Work out the finished part from the listing and answer in its coordinate system (mm). A direction names the side the tool comes from. Round coordinates to 2 decimals unless told otherwise and drop trailing zeros. Order: outer loops, then holes, each group sorted by start corner. A loop starts at its lowest first (then second) coordinate and runs counter-clockwise, first axis right, second up. Notation, with made-up numbers: (8.25, 79.5) - (46.25, 79.5) arc R26 cw to (46.25, 93.5) - close; hole circle Ø2 at (-9, -38.75). An arc over 180 degrees is marked (long way). Use CSV: the item, a comma, the result in double quotes.
from build123d import *

# Parameters (mm, degrees)
BOSS_EXTRUDE1_START = 1
SKETCH1_R           = 20
BOSS_EXTRUDE1_DEPTH = 14
FILLET2_R           = 1
CUT_EXTRUDE1_DEPTH  = 1
CUT_EXTRUDE2_START  = -2
SKETCH4_R           = 20
SKETCH4_R_2         = 19
CUT_EXTRUDE2_DEPTH  = 1
CHAMFER1_SIZE       = 1
SKETCH5_R           = 3.025
CUT_EXTRUDE3_DEPTH  = 10.5
SKETCH6_R           = 10
CUT_EXTRUDE4_DEPTH  = 5


with BuildPart() as part:
    # Sketch1 → Boss-Extrude1 (new body)
    with BuildSketch(Plane.XY.offset(BOSS_EXTRUDE1_START)):
        with Locations((51.181970815, -61.974353767)):
            Circle(SKETCH1_R)
    extrude(amount=BOSS_EXTRUDE1_DEPTH)

    # Fillet2
    fillet2_edges = [part.edges().sort_by_distance(p)[0] for p in [
        (31.181970815, -61.974353767, 15),
    ]]
    fillet(fillet2_edges, radius=FILLET2_R)

    # Sketch3 → Cut-Extrude1 (cut)
    with BuildSketch(Plane.XY.offset(15)):
        with BuildLine():
            Line((50.681970815, -61.974353767), (50.681970815, -41.974353767))
            ThreePointArc((50.681970815, -41.974353767), (51.181970815, -41.474353767), (51.681970815, -41.974353767))
            Line((51.681970815, -41.974353767), (51.681970815, -61.974353767))
            ThreePointArc((51.681970815, -61.974353767), (51.181970815, -62.474353767), (50.681970815, -61.974353767))
        make_face()
    extrude(amount=-CUT_EXTRUDE1_DEPTH, mode=Mode.SUBTRACT)

    # Sketch4 → Cut-Extrude2 (cut)
    with BuildSketch(Plane.XY.offset(15).offset(CUT_EXTRUDE2_START)):
        with Locations((51.181970815, -61.974353767)):
            Circle(SKETCH4_R)
        with Locations((51.181970815, -61.974353767)):
            Circle(SKETCH4_R_2, mode=Mode.SUBTRACT)
    extrude(amount=CUT_EXTRUDE2_DEPTH, mode=Mode.SUBTRACT)

    # Chamfer1
    chamfer1_edges = [part.edges().sort_by_distance(p)[0] for p in [
        (32.181970815, -61.974353767, 13),
    ]]
    chamfer(chamfer1_edges, length=CHAMFER1_SIZE - 0.0001)  # a hair under: the kernel refuses the full size

    # Sketch5 → Cut-Extrude3 (cut)
    with BuildSketch(Plane(origin=(0, 0, 1), x_dir=(-1, 0, 0), z_dir=(0, 0, -1))):
        with Locations((-51.181970815, -61.974353767)):
            Circle(SKETCH5_R)
    extrude(amount=-CUT_EXTRUDE3_DEPTH, mode=Mode.SUBTRACT)

    # Sketch6 → Cut-Extrude4 (cut)
    with BuildSketch(Plane(origin=(0, 0, 1), x_dir=(-1, 0, 0), z_dir=(0, 0, -1))):
        with Locations((-51.181970815, -61.974353767)):
            Circle(SKETCH6_R)
    extrude(amount=-CUT_EXTRUDE4_DEPTH, mode=Mode.SUBTRACT)


solid = part.part
(1) For faces 5 (the flat face through (51, -66, 15)), 6 (the flat face through (58, -80, 14)), 7 (the cylindrical face through (53.41, -59.93, 8.71)), 8 (the flat face through (51.682, -51.8, 14.5)), determine the directions among +Z, -Z, +X, -X, +Y, -Y from which every point of the face is accessible in a straight line to the end or side of a thin tool.
Findings below:
face 5,"+Z, +X, -X, +Y, -Y"
face 6,"none"
face 7,"-Z"
face 8,"+Z, +Y"
(2) Find section B-B (z = 2.25). Determine the outline of the cut face in (x, y).
Findings below:
outline,"circle Ø40 at (51.18, -61.97); hole circle Ø20 at (51.18, -61.97)"
(3) The mould has two halves that part along Y. Classify faces 1 (the flat face through (50.682, -52.1, 14.5)), 2 (the cylindrical face through (41.945, -65.804, 3.465)), 3 (the flat face through (54, -64, 6)), 4 (the cylindrical face through (60.41, -79.72, 6.92)): released by +Y, released by -Y, zero draft, split by the parting line, or undercut.
Findings below:
face 1,"zero draft"
face 2,"undercut"
face 3,"undercut"
face 4,"split by the parting line"
(4) Find the intervals of material crossed by L1, parallel to X at y = -63, z = 2; L2, parallel to X at y = -66, z = 2.25; L3, parallel to Z at x = 54, y = -60, in increasing order. Write a range as from..to.
Findings below:
L1,"x = 31.21..41.23, 61.13..71.16"
L2,"x = 31.59..42.03, 60.34..70.77"
L3,"z = 6..15"
(5) Find section A-A (z = 10.75). Determine the outline of the cut face in (x, y) (3 decimals), and give its area (3 significant figures).
Findings below:
outline,"circle Ø40 at (51.182, -61.974); hole circle Ø6.05 at (51.182, -61.974)"
area,"1,230 mm²"
(6) Each of these flat-tipped pins is pushed along its axis until it touches: pin 1 (4 mm diameter, centred on x = 53, y = -58.5, fed in from -Z); pin 2 (4 mm diameter, centred on x = 57.5, z = 5.5, fed in from +Y); pin 3 (3 mm diameter, centred on x = 52, y = -62, fed in from -Z). Where does it stop, or does it pass through?
Findings below:
pin 1,"stops at z = 6"
pin 2,"stops at y = -42.45"
pin 3,"stops at z = 11.5"
